Geometry: final body of the model. Coordinates: model frame, mm. A direction names the side the tool comes from. Give positions to 0.01 mm unless a question says otherwise; leave off trailing zeros. Write each loop counter-clockwise with the first axis right and the second up, starting at its lowest first coordinate (ties: lowest second). Pieces come first, ordered by that corner, then holes. Notation, with made-up numbers: M 7.5,73.5 L 27.5,73.5 A19 ccw 27.5,86.5 Z; hole C -6.75,18.5 d7. An arc over 180 degrees is marked long. Use one line per item in the form item = value. Start each with the question number.
Item 1: Access query for faces 1 (the flat face through (0, 64, 15)), 2 (the cylindrical face through (-0.1, 32.5, 9.9)). Directions: +Z, -Z, +X, -X, +Y, -Y. A direction counts if a zero-diameter tool reaches every point of the face in a straight line with its end or side. Return the directions, or none.
Item 2: Pull-direction query (X, two-part tool) for faces 3 (the cylindrical face through (-14.47, 59, 9.86)), 4 (the cylindrical face through (0, 35, 19)), 5 (the cylindrical face through (0.4, 82.5, 18.5)), 6 (the cylindrical face through (0, 85, 10)); classes: released by +X, released by -X, zero draft, split by the parting line, or undercut.
Item 3: Material intervals for line 1 along Y through (x, z) = (0, 7.75); line 2 along X through (y, z) = (40.5, 18.5); line 3 along Z through (x, y) = (7.5, 57.5), sorted ascending. Write a range as from..to.
Item 4: Contact query for flat-ended pins moving along their axis: P1, Ø12, axis at x = 28.5, y = 71, coming from the -Z side; P2, Ø4, axis at x = -21, z = 11.5, coming from the +Y side; P3, Ø2, axis at y = 55.5, z = 13.5, coming from the +X side; P4, Ø3, axis at y = 43.5, z = 5.5, coming from the +X side. Output: stop coordinate, or through.
Item 5: Section query B-B on x = 31.5. Return loops of the section in (y, z).
Item 6: Section query C-C on z = 10.5. Give the number of separate pieces and of enclosed holes in the cut face, then the cut area to 3 significant figures.
Item 7: Section query A-A on x = 0. Return loops of the section in (y, z), then the cut area to 3 significant figures.
from build123d import *

# Parameters (mm, degrees)
BOSS_EXTRUDE1_DEPTH             = 20
FILLET1_R                       = 2
RECESS_DEPTH                    = 5
RECESS_FILLET_R                 = 2
M8X1_25_TAPPED_HOLE2_AT_2_COUNT = 2
M8X1_25_TAPPED_HOLE2_AT_2_PITCH = 27


with BuildPart() as part:
    # Sketch1 → Boss-Extrude1 (new body)
    with BuildSketch(Plane.XY):
        with BuildLine():
            ThreePointArc((40.270970206, 74.854852606), (0, 85), (-40.270970206, 74.854852606))
            ThreePointArc((-40.270970206, 74.854852606), (-14.837398118, 59.604782697), (-12.374368671, 30.0520382))
            ThreePointArc((-12.374368671, 30.0520382), (0, 32.5), (12.374368671, 30.0520382))
            ThreePointArc((12.374368671, 30.0520382), (14.837398118, 59.604782697), (40.270970206, 74.854852606))
        make_face()
    extrude(amount=BOSS_EXTRUDE1_DEPTH)

    # Fillet1
    fillet1_edges = [part.edges().sort_by_distance(p)[0] for p in [
        (-12.374368671, 30.0520382, 10),
        (-40.270970206, 74.854852606, 10),
        (40.270970206, 74.854852606, 10),
        (12.374368671, 30.0520382, 10),
    ]]
    fillet(fillet1_edges, radius=FILLET1_R)

    # Sketch6 → Recess (cut)
    with BuildSketch(Plane.XY.offset(20)):
        with BuildLine():
            ThreePointArc((32.278956857, 75.923112056), (0, 82.5), (-32.278956857, 75.923112056))
            ThreePointArc((-32.278956857, 75.923112056), (-11.986412015, 59.700859487), (-8.465654652, 33.96075222))
            ThreePointArc((-8.465654652, 33.96075222), (0, 35), (8.465654652, 33.96075222))
            ThreePointArc((8.465654652, 33.96075222), (11.986412015, 59.700859487), (32.278956857, 75.923112056))
        make_face()
    extrude(amount=-RECESS_DEPTH, mode=Mode.SUBTRACT)

    # Recess Fillet
    recess_fillet_edges = [part.edges().sort_by_distance(p)[0] for p in [
        (11.986412015, 59.700859487, 15),
        (32.278956857, 75.923112056, 17.5),
        (0, 35, 15),
        (8.465654652, 33.96075222, 17.5),
        (-11.986412015, 59.700859487, 15),
        (-8.465654652, 33.96075222, 17.5),
        (0, 82.5, 15),
        (-32.278956857, 75.923112056, 17.5),
    ]]
    fillet(recess_fillet_edges, radius=RECESS_FILLET_R)

    # Sketch5 → M8x1.25 Tapped Hole2 (revolve, cut)
    with BuildSketch(Plane(origin=(0, 45, 20), x_dir=(0, -1, 0), z_dir=(1, 0, 0))):
        Polygon((0, 0), (0, 20), (4.5, 20), (3.4, 18.9), (3.4, 1.1), (4.5, 0), align=None)
    m8x1_25_tapped_hole2 = revolve(axis=Axis((0, 45, 26.35), (0, 0, -1)), mode=Mode.SUBTRACT)

    # M8x1.25 Tapped Hole2 at 2: M8x1.25 Tapped Hole2 ×2
    with Locations(*[(0, i * M8X1_25_TAPPED_HOLE2_AT_2_PITCH, 0) for i in range(1, M8X1_25_TAPPED_HOLE2_AT_2_COUNT)]):
        add(m8x1_25_tapped_hole2, mode=Mode.SUBTRACT)


solid = part.part
Answer sheet:
q1.face_1 = +Z
q1.face_2 = +Z, -Z, -Y
q2.face_3 = released by -X
q2.face_4 = undercut
q2.face_5 = undercut
q2.face_6 = split by the parting line
q3.line_1 = 32.5..41.6, 48.4..68.6, 75.4..85
q3.line_2 = -9.98..-7.48, 7.48..9.98
q3.line_3 = 0..15
q4.P1 = 0
q4.P2 = 82.85
q4.P3 = 13.13
q4.P4 = 10.03
q5.outline = M 73.03,0 L 78.95,0 L 78.95,20 L 73.03,20 Z
q6.separate_pieces = 1
q6.enclosed_holes = 2
q6.area = 1,780 mm2
q7.outline = M 32.5,0 L 40.5,0 L 41.6,1.1 L 41.6,15 L 37,15 A2 cw 35,17 L 35,20 L 32.5,20 Z; M 48.4,1.1 L 49.5,0 L 67.5,0 L 68.6,1.1 L 68.6,15 L 48.4,15 Z; M 75.4,1.1 L 76.5,0 L 85,0 L 85,20 L 82.5,20 L 82.5,17 A2 cw 80.5,15 L 75.4,15 Z
q7.area = 608 mm2
